Part model, mm, in its own coordinate system. A direction names the side the tool comes from. Round coordinates to 2 decimals unless told otherwise and drop trailing zeros. Loops run counter-clockwise (first coordinate to the right, second up) from the corner with the lowest first, then second, coordinate; pieces in that order, holes last.
(1) Cut at A-A on x = 20. List the corners of the cut face in (y, z).
(2) Cut at B-B on z = -10. List the corners of the cut face in (x, y), then the cut area to 3 significant figures.
(3) Flat gauge pins, fed straight in: pin 1 (3.5 mm diameter, centred on x = 20, y = 42.5, fed in from +Z); pin 2 (2.5 mm diameter, centred on x = 20, y = 18.5, fed in from -Z); pin 3 (0.9 mm diameter, centred on x = -35.5, z = -24.5, fed in from +Y); pin 4 (6 mm diameter, centred on x = -20, z = 0, fed in from +Y). Where does each tip first touch, or does it go through?
(4) Mould opens along X. For faces 1 (the face through (-20, 1, 1)), 2 (the face through (6, 7, -5.5)), 3 (the face through (5, 14, 0)), 4 (the face through (-15, 18.5, 0)) say: +X half, -X half, draft (parallel to the pull), parting line (faces both ways), or undercut.
(5) Cut at C-C on y = 42.5. List the corners of the cut face in (x, z), then the cut area to 3 significant figures.
(6) Probe probe 1 along Y at (x, z) = (20, -23.7); probe 2 along X at (y, z) = (3, 0); probe 3 along Z at (x, y) = (-10, 0.45). List the from-to ranges inside material, lowest first.
(7) Tool access for faces 5 (the face through (-16.806, 12.338, -1.661)), 6 (the face through (23, 30, -22.5)), 7 (the face through (-25.4, 18, -24)), 8 (the face through (-29, 13.9, -24)), 9 (the face through (-27.5, 14, 0)): list every direction of +Z, -Z, +X, -X, +Y, -Y with a clear straight run to the whole face (end or side of a thin tool).
(8) Cut at D-D on x = -26.6. List the corners of the cut face in (y, z).
from build123d import *

# Parameters (mm, degrees)
BOSS_EXTRUDE1_REACH      = 42.407
BOSS_EXTRUDE1_END_RADIUS = 5.5
SKETCH3_W                = 11
SKETCH3_H                = 18.5
SKETCH4_W                = 15
SKETCH4_H                = 50
BOSS_EXTRUDE2_DEPTH      = 20
SKETCH6_W                = 29.427394299
SKETCH6_H                = 67.669990189
CUT_EXTRUDE1_DEPTH       = 25
SKETCH5_R                = 1.3
CUT_EXTRUDE3_DEPTH       = 10
LPATTERN3_COUNT          = 3
LPATTERN3_PITCH          = 10
BOSS_EXTRUDE3_REACH      = 82.352
BOSS_EXTRUDE3_END_RADIUS = 5.5
SKETCH8_W                = 11
SKETCH8_H                = 18.5
SKETCH10_W               = 11
SKETCH10_H               = 5
BOSS_EXTRUDE4_DEPTH      = 20
SKETCH11_W               = 8.652195312
SKETCH11_H               = 5
BOSS_EXTRUDE5_DEPTH      = 20
BOSS_EXTRUDE6_DEPTH      = 20
BOSS_EXTRUDE6_DEPTH_BACK = 8.652195
SKETCH12_W               = 3
SKETCH12_H               = 50
SKETCH14_W               = 20
SKETCH14_H               = 13.9
SKETCH14_W_2             = 16.3
SKETCH14_H_2             = 21.1
CUT_EXTRUDE5_DEPTH       = 10
CHAMFER2_SIZE            = 5


with BuildPart() as part:
    # Sketch1 → Revolve1 (revolve)
    with BuildSketch(Plane.XY, mode=Mode.PRIVATE) as revolve1_sk:
        Polygon((3.6, 18.5), (5.5, 18.5), (5.5, 0), (0.5, 0), (0.5, 1), (1.2, 1), (1.2, 6), (3.6, 6), align=None)
    revolve1 = revolve(revolve1_sk.sketch.rotate(Axis((0, 0, 0), (0, 1, 0)), 90), axis=Axis((0, 0, 0), (0, 1, 0)))

    # Boss-Extrude1: up to this cylinder (the profile starts outside it)
    boss_extrude1_end = Plane(origin=(0, 9.25, 0), z_dir=(0, -1, 0)) * Cylinder(BOSS_EXTRUDE1_END_RADIUS, 96.814, mode=Mode.PRIVATE)
    # Sketch3 → Boss-Extrude1 (add, up to the surface)
    with BuildSketch(Plane(origin=(30, 0, 0), x_dir=(0, 0, -1), z_dir=(1, 0, 0)), mode=Mode.PRIVATE) as boss_extrude1_sk1:
        with Locations((0, 9.25)):
            Rectangle(SKETCH3_W, SKETCH3_H)
    boss_extrude1_tool1 = extrude(boss_extrude1_sk1.sketch, amount=-BOSS_EXTRUDE1_REACH, mode=Mode.PRIVATE) - boss_extrude1_end
    add(boss_extrude1_tool1.solids().sort_by_distance((30, 9.25, 0))[0])

    # Sketch4 → Boss-Extrude2 (add)
    with BuildSketch(Plane(origin=(0, 0, -5.5), x_dir=(-1, 0, 0), z_dir=(0, 0, -1))):
        with Locations((-22.5, 25)):
            Rectangle(SKETCH4_W, SKETCH4_H)
    extrude(amount=BOSS_EXTRUDE2_DEPTH)

    # Sketch6 → Cut-Extrude1 (cut)
    with BuildSketch(Plane(origin=(30, 0, 0), x_dir=(0, 0, -1), z_dir=(1, 0, 0))):
        with Locations((7.786302851, 38.834995095)):
            Rectangle(SKETCH6_W, SKETCH6_H)
    extrude(amount=-CUT_EXTRUDE1_DEPTH, mode=Mode.SUBTRACT)

    # Sketch5 → Cut-Extrude3 (cut)
    with BuildSketch(Plane(origin=(0, 0, -25.5), x_dir=(-1, 0, 0), z_dir=(0, 0, -1))):
        with Locations((-20, 42.5)):
            Circle(SKETCH5_R)
        with Locations((-20, 18.5)):
            Circle(SKETCH5_R)
    cut_extrude3 = extrude(amount=-CUT_EXTRUDE3_DEPTH, mode=Mode.SUBTRACT)

    # LPattern3: Revolve1 ×3
    with Locations(*[(-i * LPATTERN3_PITCH, 0, 0) for i in range(1, LPATTERN3_COUNT)]):
        add(revolve1)

    # Boss-Extrude3: up to this cylinder (the profile starts outside it)
    boss_extrude3_end = Plane(origin=(-20, 9.25, 0), z_dir=(0, -1, 0)) * Cylinder(BOSS_EXTRUDE3_END_RADIUS, 176.704, mode=Mode.PRIVATE)
    # Sketch8 → Boss-Extrude3 (add, up to the surface)
    with BuildSketch(Plane(origin=(-27.5, 0, 0), x_dir=(0, 0, -1), z_dir=(1, 0, 0)), mode=Mode.PRIVATE) as boss_extrude3_sk1:
        with Locations((0, 9.25)):
            Rectangle(SKETCH8_W, SKETCH8_H)
    boss_extrude3_tool1 = extrude(boss_extrude3_sk1.sketch, amount=BOSS_EXTRUDE3_REACH, mode=Mode.PRIVATE) - boss_extrude3_end
    add(boss_extrude3_tool1.solids().sort_by_distance((-27.5, 9.25, 0))[0])

    # Sketch10 → Boss-Extrude4 (add)
    with BuildSketch(Plane.ZY.offset(27.5)):
        with Locations((0, 2.5)):
            Rectangle(SKETCH10_W, SKETCH10_H)
    extrude(amount=BOSS_EXTRUDE4_DEPTH)

    # Sketch11 → Boss-Extrude5 (add)
    with BuildSketch(Plane(origin=(0, 0, -5.5), x_dir=(-1, 0, 0), z_dir=(0, 0, -1))):
        with Locations((43.173902344, 2.5)):
            Rectangle(SKETCH11_W, SKETCH11_H)
    extrude(amount=BOSS_EXTRUDE5_DEPTH)

    # Sketch12 → Boss-Extrude6 (add, two sides: drawn at the far end of the back side and taken through both)
    with BuildSketch(Plane(origin=(-38.847804688, 0, 0), x_dir=(0, 0, -1), z_dir=(1, 0, 0)).offset(-BOSS_EXTRUDE6_DEPTH_BACK)):
        with Locations((24, 25)):
            Rectangle(SKETCH12_W, SKETCH12_H)
    extrude(amount=BOSS_EXTRUDE6_DEPTH + BOSS_EXTRUDE6_DEPTH_BACK)

    # Mirror1: Cut-Extrude3 across plane
    add(cut_extrude3.mirror(Plane.ZY.offset(3.3)), mode=Mode.SUBTRACT)

    # Sketch14 → Cut-Extrude5 (cut)
    with BuildSketch(Plane.XY.offset(-22.5)):
        with Locations((-28.847804688, 6.95)):
            Rectangle(SKETCH14_W, SKETCH14_H)
        with Locations((-39.35, 39.45)):
            Rectangle(SKETCH14_W_2, SKETCH14_H_2)
    extrude(amount=-CUT_EXTRUDE5_DEPTH, mode=Mode.SUBTRACT)

    # Chamfer2
    chamfer2_edges = [part.edges().sort_by_distance(p)[0] for p in [
        (-27.5, 5, 0),
        (-43.173902188, 5, -22.5),
        (5, 5, 0),
        (22.5, 5, -22.5),
    ]]
    chamfer(chamfer2_edges, length=CHAMFER2_SIZE)


solid = part.part
Final values:
1. outline: (0, -25.5) - (17.2, -25.5) - (17.2, -22.5) - (10, -22.5) - (5, -17.5) - (5, 5.5) - (0, 5.5) - close; (19.8, -25.5) - (41.2, -25.5) - (41.2, -22.5) - (19.8, -22.5) - close; (43.8, -25.5) - (50, -25.5) - (50, -22.5) - (43.8, -22.5) - close
2. outline: (-47.5, 0) - (-38.85, 0) - (-38.85, 5) - (-47.5, 5) - close; (15, 0) - (30, 0) - (30, 5) - (15, 5) - close
2. area: 118 mm2
3. pin 1: stops at z = -22.5
3. pin 2: passes through
3. pin 3: stops at y = 28.9
3. pin 4: stops at y = 6
4. face 1: undercut
4. face 2: undercut
4. face 3: +X half
4. face 4: draft
5. outline: (-31.2, -25.5) - (-27.9, -25.5) - (-27.9, -22.5) - (-31.2, -22.5) - close; (-25.3, -25.5) - (-18.85, -25.5) - (-18.85, -22.5) - (-25.3, -22.5) - close; (15, -25.5) - (18.7, -25.5) - (18.7, -22.5) - (15, -22.5) - close; (21.3, -25.5) - (30, -25.5) - (30, -22.5) - (21.3, -22.5) - close
5. area: 66.5 mm2
6. probe 1: y = 0 to 17.2, 19.8 to 41.2, 43.8 to 50
6. probe 2: x = -47.5 to -21.2, -18.8 to -11.2, -8.8 to -1.2, 1.2 to 30
6. probe 3: z = -5.5 to -0.5, 0.5 to 5.5
7. face 5: +Y
7. face 6: +Z, +X, -X, +Y
7. face 7: -Z
7. face 8: -Z, -Y
7. face 9: +Z, -X, +Y
8. outline: (0, -5.5) - (18.5, -5.5) - (18.5, 5.5) - (0, 5.5) - close; (13.9, -25.5) - (17.2, -25.5) - (17.2, -22.5) - (13.9, -22.5) - close; (19.8, -25.5) - (41.2, -25.5) - (41.2, -22.5) - (19.8, -22.5) - close; (43.8, -25.5) - (50, -25.5) - (50, -22.5) - (43.8, -22.5) - close
